from build123d import *

# Parameters (mm, degrees)
SKETCH2_W                                       = 8
SKETCH2_H                                       = 8
SKETCH2_R                                       = 2
BOSS_EXTRUDE1_DEPTH                             = 7
SKETCH3_W                                       = 8
SKETCH3_H                                       = 8
BOSS_EXTRUDE2_DEPTH                             = 1
FILLET1_SIZE                                    = 2
CSK_FOR_M2_FLAT_HEAD_MACHINE_SCREW1_D           = 2.4
CSK_FOR_M2_FLAT_HEAD_MACHINE_SCREW1_DEPTH       = 7
CSK_FOR_M2_FLAT_HEAD_MACHINE_SCREW1_CSINK_D     = 4.4
CSK_FOR_M2_FLAT_HEAD_MACHINE_SCREW1_CSINK_ANGLE = 90


with BuildPart() as part:
    # Sketch2 → Boss-Extrude1 (new body)
    with BuildSketch(Plane(origin=(0, 0, 0), x_dir=(1, 0, 0), z_dir=(0, 1, 0))):
        Rectangle(SKETCH2_W, SKETCH2_H)
        with Locations(Location((0, 0, 0), (0, 0, 270))):
            Circle(SKETCH2_R, mode=Mode.SUBTRACT)
    extrude(amount=BOSS_EXTRUDE1_DEPTH)

    # Sketch3 → Boss-Extrude2 (add)
    with BuildSketch(Plane.XZ):
        Rectangle(SKETCH3_W, SKETCH3_H)
    extrude(amount=BOSS_EXTRUDE2_DEPTH)

    # Fillet1
    # a fillet whose section is not a circle: 2 mm, written as the material it takes off along each edge
    with BuildSketch(Plane(origin=(4, -6, 4), x_dir=(-1, 0, 0), z_dir=(0, 1, 0)), Plane(origin=(-4, 12, 4), x_dir=(1, 0, 0), z_dir=(0, -1, 0))) as fillet1_piece_1:
        with BuildLine():
            add(Edge.make_bspline([(FILLET1_SIZE, 0), (FILLET1_SIZE * 0.831801948466, 0), (FILLET1_SIZE * 0.663603896932, 0), (FILLET1_SIZE * 0.292893218813, -FILLET1_SIZE * 0.0716919198361), (FILLET1_SIZE * 0.0716919198361, -FILLET1_SIZE * 0.292893218813), (0, -FILLET1_SIZE * 0.663603896932), (0, -FILLET1_SIZE * 0.831801948466), (0, -FILLET1_SIZE)], knots=[0, 0, 0, 0, 0, 0, 0.5, 0.5, 1, 1, 1, 1, 1, 1], degree=5))
            Line((0, -FILLET1_SIZE), (0, 0))
            Line((0, 0), (FILLET1_SIZE, 0))
        make_face()
    extrude(amount=18, mode=Mode.SUBTRACT)
    with BuildSketch(Plane(origin=(-4, 12, -4), x_dir=(1, 0, 0), z_dir=(0, -1, 0)), Plane(origin=(4, -6, -4), x_dir=(-1, 0, 0), z_dir=(0, 1, 0))) as fillet1_piece_2:
        with BuildLine():
            add(Edge.make_bspline([(FILLET1_SIZE, 0), (FILLET1_SIZE * 0.831801948466, 0), (FILLET1_SIZE * 0.663603896932, 0), (FILLET1_SIZE * 0.292893218813, FILLET1_SIZE * 0.0716919198361), (FILLET1_SIZE * 0.0716919198361, FILLET1_SIZE * 0.292893218813), (0, FILLET1_SIZE * 0.663603896932), (0, FILLET1_SIZE * 0.831801948466), (0, FILLET1_SIZE)], knots=[0, 0, 0, 0, 0, 0, 0.5, 0.5, 1, 1, 1, 1, 1, 1], degree=5))
            Line((0, FILLET1_SIZE), (0, 0))
            Line((0, 0), (FILLET1_SIZE, 0))
        make_face()
    extrude(amount=18, mode=Mode.SUBTRACT)

    # CSK for M2 Flat Head Machine Screw1
    with Locations(Plane(origin=(0, 7, 0), x_dir=(1, 0, 0), z_dir=(0, 1, 0))):
        with Locations((0, 0)):
            CounterSinkHole(CSK_FOR_M2_FLAT_HEAD_MACHINE_SCREW1_D / 2, CSK_FOR_M2_FLAT_HEAD_MACHINE_SCREW1_CSINK_D / 2, depth=CSK_FOR_M2_FLAT_HEAD_MACHINE_SCREW1_DEPTH, counter_sink_angle=CSK_FOR_M2_FLAT_HEAD_MACHINE_SCREW1_CSINK_ANGLE)


solid = part.part
Read the model definition and answer for the solid it produces. Units are mm, in the model's axes. Round coordinates to 2 decimals unless told otherwise and drop trailing zeros. Loops run counter-clockwise (first coordinate to the right, second up) from the corner with the lowest first, then second, coordinate; pieces in that order, holes last.
Q1. Consider probe 1 along Z at (x, y) = (0, 1.5); probe 2 along X at (y, z) = (0.75, -1.25). Determine where each line is inside the solid, lowest interval first.
Q2. This flat-tipped pin is pushed along its axis until it touches: pin 1 (3 mm diameter, centred on y = 5, z = -3, fed in from -X). Where does it stop, or does it pass through?
Q3. Section A-A on z = 0 is taken. Write down the section's boundary in (x, y), and give its area (3 significant figures).
Q4. Determine the mould class of faces 1 (the face through (0, 0, 0)), 2 (the face through (0, 3, 4)), 3 (the face through (4, 3, 0)), 4 (the face through (-2, 3, 0)) for opening direction X: released by +X, released by -X, zero draft, split by the parting line, or undercut.
Q5. Section B-B on x = 0 is taken. Write down the section's boundary in (y, z), and give its area (3 significant figures).
Output:
1. probe 1: z = -4 to -2, 2 to 4
1. probe 2: x = -4 to -1.56, 1.56 to 4
2. pin 1: stops at x = -4
3. outline: (-4, -1) - (4, -1) - (4, 7) - (2.2, 7) - (2, 6.8) - (2, 0) - (-2, 0) - (-2, 6.8) - (-2.2, 7) - (-4, 7) - close
3. area: 36.0 mm2
4. face 1: undercut
4. face 2: zero draft
4. face 3: released by +X
4. face 4: undercut
5. outline: (-1, -4) - (7, -4) - (7, -2.2) - (6.8, -2) - (0, -2) - (0, 2) - (6.8, 2) - (7, 2.2) - (7, 4) - (-1, 4) - close
5. area: 36.0 mm2
